```python
from build123d import *

# Parameters (mm, degrees)
ESBO_O1_W                = 150
ESBO_O1_H                = 100
ESBO_O1_R                = 6.5
ESBO_O1_R_2              = 1.5
RESSALTO_EXTRUS_O1_DEPTH = 3


with BuildPart() as part:
    # Esboço1 → Ressalto-extrusão1 (new body)
    with BuildSketch(Plane.XY):
        with Locations((75, 50)):
            Rectangle(ESBO_O1_W, ESBO_O1_H)
        with Locations((75, 75)):
            Circle(ESBO_O1_R, mode=Mode.SUBTRACT)
        with Locations((104.5, 86)):
            Circle(ESBO_O1_R_2, mode=Mode.SUBTRACT)
        with Locations(Location((104.5, 64, 0), (0, 0, 180))):
            Circle(ESBO_O1_R_2, mode=Mode.SUBTRACT)
        with Locations((45.5, 64)):
            Circle(ESBO_O1_R_2, mode=Mode.SUBTRACT)
        with Locations(Location((45.5, 86, 0), (0, 0, 180))):
            Circle(ESBO_O1_R_2, mode=Mode.SUBTRACT)
    extrude(amount=RESSALTO_EXTRUS_O1_DEPTH)


solid = part.part
```
Can you work these out from the model? Positions are in its coordinate system, mm. Coordinates: 2 decimals unless noted, no trailing zeros. Order: outer loops, then holes, each group sorted by start corner. A loop starts at its lowest first (then second) coordinate and runs counter-clockwise, first axis right, second up.
1. I'm going to push a flat-ended pin straight in: pin 1 (2.5 mm diameter, centred on x = 104.5, y = 64, fed in from +Z). Where does the tip first touch, or does it pass through?
2. If we section it at D-D (y = 75): Please give me the cut outline in (x, z), then the cut area to 3 significant figures.
3. If we section it at A-A (x = 75): Please give me the cut outline in (y, z), then the cut area to 3 significant figures.
4. If we section it at B-B (y = 64): Please give me the cut outline in (x, z).
5. I need wall thicknesses on line 1 (X direction, y = 86, z = 1.7); line 2 (Y direction, x = 104.5, z = 1.75); line 3 (Y direction, x = 73.5, z = 2.25). Which ranges of each line are inside material? Lowest first, please.
6. Thinking about a two-plate mould opening in Y: for faces 1 (the face through (150, 49, 1)), 2 (the face through (105.61, 62.99, 1.48)), 3 (the face through (46.61, 84.99, 1.48)), 4 (the face through (74, 0, 1)), which applies, +Y half, -Y half, draft (parallel to the pull), parting line (faces both ways), or undercut?
7. If we section it at C-C (x = 45.5): Please give me the cut outline in (y, z).
Entries:
1. pin 1: passes through
2. outline: (0, 0) - (68.5, 0) - (68.5, 3) - (0, 3) - close; (81.5, 0) - (150, 0) - (150, 3) - (81.5, 3) - close
2. area: 411 mm2
3. outline: (0, 0) - (68.5, 0) - (68.5, 3) - (0, 3) - close; (81.5, 0) - (100, 0) - (100, 3) - (81.5, 3) - close
3. area: 261 mm2
4. outline: (0, 0) - (44, 0) - (44, 3) - (0, 3) - close; (47, 0) - (103, 0) - (103, 3) - (47, 3) - close; (106, 0) - (150, 0) - (150, 3) - (106, 3) - close
5. line 1: x = 0 to 44, 47 to 103, 106 to 150
5. line 2: y = 0 to 62.5, 65.5 to 84.5, 87.5 to 100
5. line 3: y = 0 to 68.68, 81.32 to 100
6. face 1: draft
6. face 2: undercut
6. face 3: undercut
6. face 4: -Y half
7. outline: (0, 0) - (62.5, 0) - (62.5, 3) - (0, 3) - close; (65.5, 0) - (84.5, 0) - (84.5, 3) - (65.5, 3) - close; (87.5, 0) - (100, 0) - (100, 3) - (87.5, 3) - close
